Geometry: final body of the model. Coordinates: model frame, mm. A direction names the side the tool comes from. Round coordinates to 2 decimals unless told otherwise and drop trailing zeros. Loops run counter-clockwise (first coordinate to the right, second up) from the corner with the lowest first, then second, coordinate; pieces in that order, holes last. Notation, with made-up numbers: (11, 52.25) -> (15, 52.25) arc R27 cw to (15, 76.25) -> close; hole circle Ø1 at (79.5, 77.5). An arc over 180 degrees is marked (long way). Answer in a Markdown table with one row per item.
```python
from build123d import *

# Parameters (mm, degrees)
SKETCH1_R           = 1.6
BOSS_EXTRUDE1_DEPTH = 3
CUT_EXTRUDE1_DEPTH  = 3
FILLET1_R           = 3
CUT_EXTRUDE2_DEPTH  = 47.615448083
FILLET2_R           = 2


with BuildPart() as part:
    # Sketch1 → Boss-Extrude1 (new body)
    with BuildSketch(Plane(origin=(0, 53, 0), x_dir=(1, 0, 0), z_dir=(0, 1, 0))):
        with BuildLine():
            Line((-37, 20), (37, 20))
            ThreePointArc((37, 20), (40.535533906, 18.535533906), (42, 15))
            Line((42, 15), (42, -15))
            ThreePointArc((42, -15), (40.535533906, -18.535533906), (37, -20))
            Line((37, -20), (-37, -20))
            ThreePointArc((-37, -20), (-40.535533906, -18.535533906), (-42, -15))
            Line((-42, -15), (-42, 15))
            ThreePointArc((-42, 15), (-40.535533906, 18.535533906), (-37, 20))
        make_face()
        with Locations(Location((37, 14.944086969, 0), (0, 0, 270))):
            Circle(SKETCH1_R, mode=Mode.SUBTRACT)
        with Locations(Location((37, -14.944086969, 0), (0, 0, 270))):
            Circle(SKETCH1_R, mode=Mode.SUBTRACT)
        with Locations(Location((-37, -15, 0), (0, 0, 270))):
            Circle(SKETCH1_R, mode=Mode.SUBTRACT)
        with Locations(Location((-37, 15, 0), (0, 0, 270))):
            Circle(SKETCH1_R, mode=Mode.SUBTRACT)
    extrude(amount=BOSS_EXTRUDE1_DEPTH)

    # Sketch2 → Cut-Extrude1 (cut)
    with BuildSketch(Plane(origin=(0, 56, 0), x_dir=(1, 0, 0), z_dir=(0, 1, 0))):
        Polygon((-27, 20), (-24.113248654, 15), (19.859259966, 15), (27, 20), align=None)
        Polygon((-27, -20), (27, -20), (19.859259966, -15), (-24.113248654, -15), align=None)
        with BuildLine():
            Line((42, 11), (42, -11))
            ThreePointArc((42, -11), (34.795831523, 0), (42, 11))
        make_face()
        with BuildLine():
            Line((-42, 8), (-42, -8))
            ThreePointArc((-42, -8), (-34, 0), (-42, 8))
        make_face()
    extrude(amount=-CUT_EXTRUDE1_DEPTH, mode=Mode.SUBTRACT)

    # Fillet1
    fillet1_edges = [part.edges().sort_by_distance(p)[0] for p in [
        (-24.113248654, 54.5, -15),
        (19.859259966, 54.5, -15),
        (27, 54.5, -20),
        (-27, 54.5, -20),
        (27, 54.5, 20),
        (19.859259966, 54.5, 15),
        (-24.113248654, 54.5, 15),
        (-27, 54.5, 20),
    ]]
    fillet(fillet1_edges, radius=FILLET1_R)

    # Sketch3 → Cut-Extrude2 (cut, through all)
    with BuildSketch(Plane(origin=(0, 56, 0), x_dir=(1, 0, 0), z_dir=(0, 1, 0))):
        Polygon((20.863248654, 0), (16.244446501, 8), (19.131197846, 8), (23.75, 0), (19.131197846, -8), (16.244446501, -8), align=None)
        Polygon((10.863248654, 0), (6.244446501, 8), (9.131197846, 8), (13.75, 0), (9.131197846, -8), (6.244446501, -8), align=None)
        Polygon((0.863248654, 0), (-3.755553499, 8), (-0.868802154, 8), (3.75, 0), (-0.868802154, -8), (-3.755553499, -8), align=None)
        Polygon((-9.136751346, 0), (-13.755553499, 8), (-10.868802154, 8), (-6.25, 0), (-10.868802154, -8), (-13.755553499, -8), align=None)
        Polygon((-19.136751346, 0), (-23.755553499, 8), (-20.868802154, 8), (-16.25, 0), (-20.868802154, -8), (-23.755553499, -8), align=None)
    extrude(amount=-CUT_EXTRUDE2_DEPTH, mode=Mode.SUBTRACT)

    # Fillet2
    fillet2_edges = [part.edges().sort_by_distance(p)[0] for p in [
        (42, 54.5, -11),
        (42, 54.5, 11),
        (-42, 54.5, 8),
        (-42, 54.5, -8),
    ]]
    fillet(fillet2_edges, radius=FILLET2_R)


solid = part.part
```
Item 1: First-contact query: P1, Ø1.4, axis at x = 17, y = 55, coming from the -Z side; P2, Ø0.9, axis at x = -13, y = 54.5, coming from the +Z side; P3, Ø1, axis at x = -23, y = 53.5, coming from the -Z side. Flat tips, straight axial feed; report the tip coordinate or a pass-through.
Ans:
| item | result |
|---|---|
| P1 | z = -15 |
| P2 | z = 15 |
| P3 | z = -15.22 |
Item 2: Section query D-D, the plane z = -9. Output: boundary loops of the cut face in (x, y), and give its area (3 significant figures).
Ans:
| item | result |
|---|---|
| outline | (-41.83, 53) -> (38.86, 53) -> (38.86, 56) -> (-41.83, 56) -> close |
| area | 242 mm2 |
Item 3: Section query C-C, the plane y = 55. State how many separate pieces and enclosed holes the cut face has, and give its area (3 significant figures).
Ans:
| item | result |
|---|---|
| separate pieces | 1 |
| enclosed holes | 9 |
| area | 2,370 mm2 |
Item 4: Section query A-A, the plane x = 3. Output: boundary loops of the cut face in (y, z).
Ans:
| item | result |
|---|---|
| outline | (53, -15) -> (56, -15) -> (56, -1.3) -> (53, -1.3) -> close; (53, 1.3) -> (56, 1.3) -> (56, 15) -> (53, 15) -> close |
Item 5: Section query B-B, the plane z = 2.5. Output: boundary loops of the cut face in (x, y).
Ans:
| item | result |
|---|---|
| outline | (-34.4, 53) -> (-20.58, 53) -> (-20.58, 56) -> (-34.4, 56) -> close; (-17.69, 53) -> (-10.58, 53) -> (-10.58, 56) -> (-17.69, 56) -> close; (-7.69, 53) -> (-0.58, 53) -> (-0.58, 56) -> (-7.69, 56) -> close; (2.31, 53) -> (9.42, 53) -> (9.42, 56) -> (2.31, 56) -> close; (12.31, 53) -> (19.42, 53) -> (19.42, 56) -> (12.31, 56) -> close; (22.31, 53) -> (35.06, 53) -> (35.06, 56) -> (22.31, 56) -> close |
Item 6: Mould query, pull axis X, two halves, no side actions, for faces 1 (the flat face through (1, 53, 9)), 2 (the cylindrical face through (27.032, 54.479, 19.857)), 3 (the flat face through (-12, 55, -8)), 4 (the cylindrical face through (-41, 54, -18)). Classes: released by +X, released by -X, zero draft, split by the parting line, or undercut.
Ans:
| item | result |
|---|---|
| face 1 | zero draft |
| face 2 | undercut |
| face 3 | undercut |
| face 4 | released by -X |
Item 7: Set-up query: faces 5 (the cylindrical face through (19.828, 54.479, -15.143)), 6 (the flat face through (8.59, 54.52, -3.94)), 7 (the flat face through (-1, 55, 15)), 8 (the cylindrical face through (41.73, 54.48, 11.24)). Return all of +Z, -Z, +X, -X, +Y, -Y with unobstructed straight access to the full face (end or side cutting, diameter ignored); none if empty.
Ans:
| item | result |
|---|---|
| face 5 | -Z, +Y, -Y |
| face 6 | +Y, -Y |
| face 7 | +Z, +Y, -Y |
| face 8 | +X, +Y, -Y |
Item 8: Ray query, L1, parallel to Z at x = -20.5, y = 55.8; L2, parallel to X at y = 54.55, z = 16; L3, parallel to X at y = 54.15, z = 7. Return the intervals inside material, ascending.
Ans:
| item | result |
|---|---|
| L1 | -15 to -7.36, -2.36 to 2.36, 7.36 to 15 |
| L2 | -41.9 to -38.25, -35.75 to -24.62, 21.29 to 35.8, 38.2 to 41.9 |
| L3 | -38.13 to -23.18, -20.29 to -13.18, -10.29 to -3.18, -0.29 to 6.82, 9.71 to 16.82, 19.71 to 37.05 |
